Input: part model. Units: mm. Frame: model coordinates. Face numbers are marked on the shaded views. A direction names the side the tool comes from. Give positions to 0.01 mm unless a question says otherwise; leave off trailing zeros. Write each loop counter-clockwise with the first axis right and the second up, starting at its lowest first coordinate (ties: lowest second). Pieces come first, ordered by that corner, then holes.
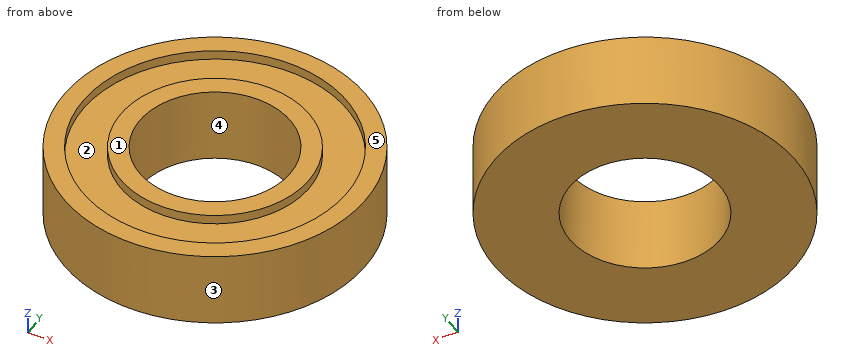
```python
from build123d import *

# Parameters (mm, degrees)
SKETCH016_R     = 8
SKETCH016_R_2   = 4
PAD009_DEPTH    = 4
SKETCH017_R     = 7
SKETCH017_R_2   = 5
POCKET008_DEPTH = 0.5
SKETCH018_R     = 20
SKETCH018_R_2   = 16
POCKET009_DEPTH = 0.5


with BuildPart() as part:
    # Sketch016 → Pad009 (new body)
    with BuildSketch(Plane.XY):
        Circle(SKETCH016_R)
        Circle(SKETCH016_R_2, mode=Mode.SUBTRACT)
    extrude(amount=PAD009_DEPTH)

    # Sketch017 → Pocket008 (cut)
    with BuildSketch(Plane.XY.offset(4)):
        Circle(SKETCH017_R)
        Circle(SKETCH017_R_2, mode=Mode.SUBTRACT)
    extrude(amount=-POCKET008_DEPTH, mode=Mode.SUBTRACT)

    # Sketch018 → Pocket009 (cut)
    with BuildSketch(Plane.XY):
        Circle(SKETCH018_R)
        Circle(SKETCH018_R_2, mode=Mode.SUBTRACT)
    extrude(amount=POCKET009_DEPTH, mode=Mode.SUBTRACT)


solid = part.part
```
Item 1: Set-up query: the marked faces 1 and 2. Return all of +Z, -Z, +X, -X, +Y, -Y with unobstructed straight access to the full face (end or side cutting, diameter ignored); none if empty.
Item 2: Mould query, pull axis X, two halves, no side actions, for the marked faces 3, 4 and 5. Classes: +X half, -X half, draft (parallel to the pull), parting line (faces both ways), or undercut.
Item 3: Ray query, line 1 (Y direction, x = 0, z = 3.8); line 2 (Y direction, x = 0, z = 2.3); line 3 (X direction, y = -1, z = 3.65). Return the intervals inside material, ascending.
Item 4: Pin query (flat end, axial travel): pin 1 (6 mm diameter, centred on x = -4.5, y = -3, fed in from +Z); pin 2 (1 mm diameter, centred on x = 5, z = 1.5, fed in from +Y); pin 3 (1.5 mm diameter, centred on x = -3, z = 3.5, fed in from +Y); pin 4 (7 mm diameter, centred on x = 0, y = 0, fed in from +Z). Return the tip coordinate at first contact, or that it passes through.
Item 5: Section C-C (z = 0.9). Return loops of the section in (x, y).
Item 6: Section A-A (x = 0). Return loops of the section in (y, z), and give its area (3 significant figures).
Solved:
1. face 1: +Z, +X, -X, +Y, -Y
1. face 2: +Z
2. face 3: parting line
2. face 4: undercut
2. face 5: draft
3. line 1: y = -8 to -7, -5 to -4, 4 to 5, 7 to 8
3. line 2: y = -8 to -4, 4 to 8
3. line 3: x = -7.94 to -6.93, -4.9 to -3.87, 3.87 to 4.9, 6.93 to 7.94
4. pin 1: stops at z = 4
4. pin 2: stops at y = 6.61
4. pin 3: stops at y = 7.68
4. pin 4: passes through
5. outline: circle Ø16 at (0, 0); hole circle Ø8 at (0, 0)
6. outline: (-8, 0) - (-4, 0) - (-4, 4) - (-5, 4) - (-5, 3.5) - (-7, 3.5) - (-7, 4) - (-8, 4) - close; (4, 0) - (8, 0) - (8, 4) - (7, 4) - (7, 3.5) - (5, 3.5) - (5, 4) - (4, 4) - close
6. area: 30.0 mm2
